Autodesk Inventor part; units mm, degrees
ref_plane "YZ Plane" through (0, 0, 0) normal (1, 0, 0) x (0, 1, 0)
ref_plane "XZ Plane" through (0, 0, 0) normal (0, 1, 0) x (-1, 0, 0)
ref_plane "XY Plane" through (0, 0, 0) normal (0, 0, 1) x (1, 0, 0)
sketch "Sketch1" plane through (0, 0, 0) normal (0, 0, 1) x (1, 0, 0)
  line L0 (0, 0) -> (0, -38.1)
  line L1 (0, -38.1) -> (1219.2, -38.1)
  line L2 (1219.2, 0) -> (1219.2, -38.1)
  line L3 (0, 0) -> (1219.2, 0)
  line L4 (0, 0) -> (914.4, 0)
  line L5 (914.4, 609.6) -> (0, 0)
  line L6 (914.4, 609.6) -> (1219.2, 0)
  line L7 (1219.2, 0) -> (1126.19, 0)
  line L8 (1119.8068, 0) -> (879.9218, 479.77)
  line L9 (1119.8068, 0) -> (1219.2, 0)
  line L10 (160.2668, 0) -> (879.9218, 479.77)
  line L11 (879.9218, 479.77) -> (954.4667, 529.4666)
  dimension "d3" = 88.9
extrude "Extrusion1" add sketch "Sketch1" against normal blind 38.1 contours L5 L6 L11 L10 L3
properties part number "S_2x4x43.267"
Source: CAD feature listing. Evaluate the final solid. Frame: model axes, mm. Round coordinates to 2 decimals unless told otherwise and drop trailing zeros. Order: outer loops, then holes, each group sorted by start corner. A loop starts at its lowest first (then second) coordinate and runs counter-clockwise, first axis right, second up. Notation, with made-up numbers: (17.5, 42.25) - (68.5, 42.25) arc R29 ccw to (68.5, 79.25) - close; hole circle Ø5 at (86, 83.25). An arc over 180 degrees is marked (long way). Use a Markdown table: item, result. Add a question column.
1. Section query B-B (x = 483.5). Return the cut outline in (y, z), then the cut area to 3 significant figures.
2. Section query A-A (z = -11). Return the cut outline in (x, y), then the cut area to 3 significant figures.
3. Line query: probe 1 along Y at (x, z) = (608.5, -31); probe 2 along Y at (x, z) = (856, -11); probe 3 along X at (y, z) = (367, -33). Output: solid intervals per line, ascending.
4. First-contact query: pin 1 (6 mm diameter, centred on x = 752, z = -34, fed in from +Y); pin 2 (4 mm diameter, centred on x = 486, z = -32.5, fed in from +Y); pin 3 (10 mm diameter, centred on y = 291.5, z = -29, fed in from +X). Flat tips, straight axial feed; report the tip coordinate or a pass-through.
Derived:
| question | item | result |
|---|---|---|
| 1 | outline | (215.49, -38.1) - (322.33, -38.1) - (322.33, 0) - (215.49, 0) - close |
| 1 | area | 4,070 mm2 |
| 2 | outline | (0, 0) - (160.27, 0) - (954.47, 529.47) - (914.4, 609.6) - close |
| 2 | area | 91,300 mm2 |
| 3 | probe 1 | 298.82 to 405.67 |
| 3 | probe 2 | 463.82 to 570.67 |
| 3 | probe 3 | 550.5 to 710.77 |
| 4 | pin 1 | y = 503.33 |
| 4 | pin 2 | y = 325.33 |
| 4 | pin 3 | x = 605.02 |
